Read the model definition and answer for the solid it produces. Units are mm, in the model's axes. Give positions to 0.01 mm unless a question says otherwise; leave off trailing zeros. Write each loop counter-clockwise with the first axis right and the second up, starting at its lowest first coordinate (ties: lowest second). Pieces come first, ordered by that corner, then holes. Notation, with made-up numbers: M -5,49.25 L 3,49.25 A27 ccw 3,88.25 Z; hole C 34.5,76 d4. An arc over 180 degrees is marked long. Write each question's results on one line, items separated by ' | '. Start each with the question number.
```python
from build123d import *

# Parameters (mm, degrees)
F1_DEPTH = 7.28025


with BuildPart() as f1:
    # F0 (on Top) → F1 (new body)
    with BuildSketch(Plane.XY):
        with BuildLine():
            ThreePointArc((-2.3495, 0), (12.985089, -11.099056), (18.737294, 6.935655))
            Line((18.737294, 6.935655), (14.574847, 12.664773))
            ThreePointArc((14.574847, 12.664773), (13.788343, 13.082964), (12.974584, 12.720656))
            Line((12.974584, 12.720656), (10.545117, 9.82533))
            ThreePointArc((10.545117, 9.82533), (10.158151, 7.994524), (11.462635, 6.652914))
            ThreePointArc((11.462635, 6.652914), (13.453068, -5.641598), (2.3495, 0))
            ThreePointArc((2.3495, 0), (0, 2.3495), (-2.3495, 0))
        make_face()
    extrude(amount=F1_DEPTH)


solid = f1.part
```
Item 1: Section C-C, the plane x = 15.25 is taken. Determine the outline of the cut face in (y, z).
Item 2: Section B-B, the plane y = -0.75 is taken. Determine the outline of the cut face in (x, z).
Item 3: Straight lines are drawn through the part: line 1 (X direction, y = 0, z = 2.25); line 2 (X direction, y = -6.25, z = 6.25); line 3 (Y direction, x = 13.75, z = 0.75). For each, find the intervals that lie inside material, in ascending order.
Item 4: Determine the mould class of faces 1 (the cylindrical face through (10.15, 8.02, 3.59)), 2 (the flat face through (16.685, 9.76, 3.589)), 3 (the flat face through (12, -7, 0)), 4 (the cylindrical face through (13.625, -5.512, 3.589)) for opening direction Y: +Y half, -Y half, draft (parallel to the pull), parting line (faces both ways), or undercut.
Item 5: Section D-D, the plane x = 0 is taken. Determine the outline of the cut face in (y, z), then the cut area to 3 significant figures.
Item 6: Given P1, Ø2, axis at y = 7, z = 3.5, coming from the -X side; P2, Ø1.5, axis at x = 16, z = 6.5, coming from the +Y side; P3, Ø1, axis at y = -6.5, z = 3, coming from the -X side, each flat-ended and moving along its own axis, determine where each tip first touches the part or whether it passes through.
Item 7: Section A-A, the plane z = 2 is taken. Determine the outline of the cut face in (x, y) (1 decimal).
Worked out:
1) outline: M -10.08,0 L -3.71,0 L -3.71,7.28 L -10.08,7.28 Z; M 3.71,0 L 11.74,0 L 11.74,7.28 L 3.71,7.28 Z
2) outline: M -2.33,0 L 2.39,0 L 2.39,7.28 L -2.33,7.28 Z; M 16.28,0 L 20.99,0 L 20.99,7.28 L 16.28,7.28 Z
3) line 1: x = -2.35 to 2.35, 16.32 to 21.02 | line 2: x = -0.54 to 6.22, 12.45 to 19.21 | line 3: y = -10.82 to -5.41, 5.41 to 13.08
4) face 1: undercut | face 2: +Y half | face 3: draft | face 4: undercut
5) outline: M -7.03,0 L 2.35,0 L 2.35,7.28 L -7.03,7.28 Z | area: 68.3 mm²
6) P1: stops at x = 10.16 | P2: stops at y = 11.74 | P3: stops at x = -0.69
7) outline: M -2.3,0 A11.7 ccw long 18.7,6.9 L 14.6,12.7 A1 ccw 13,12.7 L 10.5,9.8 A2 ccw 11.5,6.7 A7 cw long 2.3,0 A2.3 ccw Z
